For this review, take the finished solid that the model builds, in its own axes (mm). A direction names the side the tool comes from. Give positions to 0.01 mm unless a question says otherwise; leave off trailing zeros. Write each loop counter-clockwise with the first axis right and the second up, starting at its lowest first coordinate (ties: lowest second). Pieces come first, ordered by that corner, then holes. Notation, with made-up numbers: (-33.75, -9.5) -> (24.25, -9.5) arc R34 cw to (24.25, 28.5) -> close; hole circle Ø5 at (-15, -0.75). An arc over 180 degrees is marked (long way). Answer as CSV lines item,"result".
```python
from build123d import *

# Parameters (mm, degrees)
SKETCH1_W          = 84.836
SKETCH1_H          = 69.342
BASE_FLANGE1_DEPTH = 4.826
SKETCH6_R          = 2.54
CUT_EXTRUDE1_DEPTH = 10
FILLET1_R          = 2.6
SKETCH7_W          = 18.5
SKETCH7_H          = 10
SKETCH7_W_2        = 43
SKETCH7_H_2        = 5
SKETCH7_W_3        = 7
CUT_EXTRUDE2_DEPTH = 4.826
FILLET2_R          = 2.4
FILLET3_R          = 1.6


# Sheet-metal steps are written as plain solids
with BuildPart() as part:
    # Sketch1 → Base-Flange1 (new body)
    with BuildSketch(Plane.XY):
        Rectangle(SKETCH1_W, SKETCH1_H)
    extrude(amount=-BASE_FLANGE1_DEPTH)

    # Sketch6 → Cut-Extrude1 (cut)
    with BuildSketch(Plane.XY):
        with Locations((-37.846, 30.099)):
            Circle(SKETCH6_R)
        with Locations(Location((-37.846, -30.099, 0), (0, 0, 180))):
            Circle(SKETCH6_R)
        with Locations((37.846, -30.099)):
            Circle(SKETCH6_R)
        with Locations(Location((37.846, 30.099, 0), (0, 0, 180))):
            Circle(SKETCH6_R)
    extrude(amount=-CUT_EXTRUDE1_DEPTH, mode=Mode.SUBTRACT)

    # Fillet1
    fillet1_edges = [part.edges().sort_by_distance(p)[0] for p in [
        (-42.418, 34.671, -2.413),
        (42.418, 34.671, -2.413),
        (42.418, -34.671, -2.413),
        (-42.418, -34.671, -2.413),
    ]]
    fillet(fillet1_edges, radius=FILLET1_R)

    # Sketch7 → Cut-Extrude2 (cut)
    with BuildSketch(Plane.XY):
        with Locations((-33.168, 18.7119922)):
            Rectangle(SKETCH7_W, SKETCH7_H)
        Polygon((-42.418, -4.5120046), (-26.418, -4.5120046), (-26.418, -26.512012), (-35.418, -26.512012), (-35.418, -17.5120046), (-42.418, -17.5120046), align=None)
        with Locations((9.2919882, 24.3120114)):
            Rectangle(SKETCH7_W_2, SKETCH7_H_2)
        Polygon((-14.2080118, -21.81200997), (-14.2080118, -16.31199997), (-23.2080118, -16.31199997), (-23.2080118, -26.81199997), (30.7919882, -26.81199997), (30.7919882, -21.81200997), align=None)
        with Locations((27.8920124, 1.371)):
            Rectangle(SKETCH7_W_3, SKETCH7_H)
    extrude(amount=-CUT_EXTRUDE2_DEPTH, mode=Mode.SUBTRACT)

    # Fillet2
    fillet2_edges = [part.edges().sort_by_distance(p)[0] for p in [
        (-12.2080118, 21.8120114, -2.413),
        (-12.2080118, 26.8120114, -2.413),
        (30.7919882, 26.8120114, -2.413),
        (30.7919882, 21.8120114, -2.413),
        (30.7919882, -21.81200997, -2.413),
        (30.7919882, -26.81199997, -2.413),
        (-23.2080118, -26.81199997, -2.413),
        (-14.2080118, -21.81200997, -2.413),
        (-26.418, -26.512012, -2.413),
        (-35.418, -26.512012, -2.413),
    ]]
    fillet(fillet2_edges, radius=FILLET2_R)

    # Fillet3
    fillet3_edges = [part.edges().sort_by_distance(p)[0] for p in [
        (24.3920124, -3.629, -2.413),
        (24.3920124, 6.371, -2.413),
        (31.3920124, 6.371, -2.413),
        (31.3920124, -3.629, -2.413),
        (-23.2080118, -16.31199997, -2.413),
        (-14.2080118, -16.31199997, -2.413),
        (-23.918, 23.7119922, -2.413),
        (-23.918, 13.7119922, -2.413),
        (-26.418, -4.5120046, -2.413),
    ]]
    fillet(fillet3_edges, radius=FILLET3_R)


solid = part.part
```
Q1. Add section B-B (y = -1). Write out the cut boundary in (x, z), plus the area to 3 significant figures.
Answer block:
outline,"(-42.42, -4.83) -> (24.39, -4.83) -> (24.39, 0) -> (-42.42, 0) -> close; (31.39, -4.83) -> (42.42, -4.83) -> (42.42, 0) -> (31.39, 0) -> close"
area,"376 mm2"
Q2. Add section A-A (x = -2.5). Write out the cut boundary in (y, z), plus the area to 3 significant figures.
Answer block:
outline,"(-34.67, -4.83) -> (-26.81, -4.83) -> (-26.81, 0) -> (-34.67, 0) -> close; (-21.81, -4.83) -> (21.81, -4.83) -> (21.81, 0) -> (-21.81, 0) -> close; (26.81, -4.83) -> (34.67, -4.83) -> (34.67, 0) -> (26.81, 0) -> close"
area,"286 mm2"
Q3. For faces 1 (the cylindrical face through (-22.524, -26.09, -2.447)), 2 (the flat face through (-39, -17.512, -2)), 3 (the flat face through (42.418, 0, -2)), list the 3-axis set-ups (+Z, -Z, +X, -X, +Y, -Y) from which the entire face can be reached by the end or side of a thin tool; tool diameter is ignored.
Answer block:
face 1,"+Z, -Z"
face 2,"+Z, -Z, -X"
face 3,"+Z, -Z, +X, +Y, -Y"
Q4. Draft analysis for pull direction Y (two halves, no side actions). For faces 4 (the flat face through (-42.418, 28, -2)), 5 (the flat face through (-1, -34.671, -2)), 6 (the flat face through (-1, 34.671, -2)), 7 (the flat face through (-23.208, -21, -2)), state which applies: released by +Y, released by -Y, zero draft, split by the parting line, or undercut.
Answer block:
face 4,"zero draft"
face 5,"released by -Y"
face 6,"released by +Y"
face 7,"undercut"
Q5. Clearance check with a flat-ended pin moving along its axis: pin 1 (6 mm diameter, centred on x = 3.5, y = 13, fed in from +Z). State where the tip first meets the part, or that it passes through.
Answer block:
pin 1,"stops at z = 0"
Q6. To check wall thickness, follow probe 1 along Y at (x, z) = (-31.5, -1.3); probe 2 along Y at (x, z) = (9, -2.35); probe 3 along X at (y, z) = (-2, -2.1). State the ranges of each line that lie inside material, in increasing order. Write a range as [from, to].
Answer block:
probe 1,"y = [-34.67, -26.51], [-4.51, 13.71], [23.71, 34.67]"
probe 2,"y = [-34.67, -26.81], [-21.81, 21.81], [26.81, 34.67]"
probe 3,"x = [-42.42, 24.39], [31.39, 42.42]"
Q7. Add section D-D (z = -2.75). State how many separate pieces and enclosed holes the cut face has, plus the area to 3 significant figures.
Answer block:
separate pieces,"1"
enclosed holes,"7"
area,"4,730 mm2"
Q8. Add section C-C (y = -23). Write out the cut boundary in (x, z).
Answer block:
outline,"(-42.42, -4.83) -> (-35.42, -4.83) -> (-35.42, 0) -> (-42.42, 0) -> close; (-26.42, -4.83) -> (-23.21, -4.83) -> (-23.21, 0) -> (-26.42, 0) -> close; (30.46, -4.83) -> (42.42, -4.83) -> (42.42, 0) -> (30.46, 0) -> close"
